```python
from build123d import *

# Parameters (mm, degrees)
SKETCH1_W           = 1.5
SKETCH1_H           = 3
BOSS_EXTRUDE1_DEPTH = 5


with BuildPart() as part:
    # Sketch1 → Boss-Extrude1 (new body)
    with BuildSketch(Plane(origin=(0, 0, 0), x_dir=(1, 0, 0), z_dir=(0, 1, 0))):
        Rectangle(SKETCH1_W, SKETCH1_H)
        Polygon((0.75, 6), (0.75, 1.5), (-0.75, 1.5), (-0.75, 7.5), (0.75, 7.5), (2.25, 6), align=None)
    extrude(amount=BOSS_EXTRUDE1_DEPTH)


solid = part.part
```
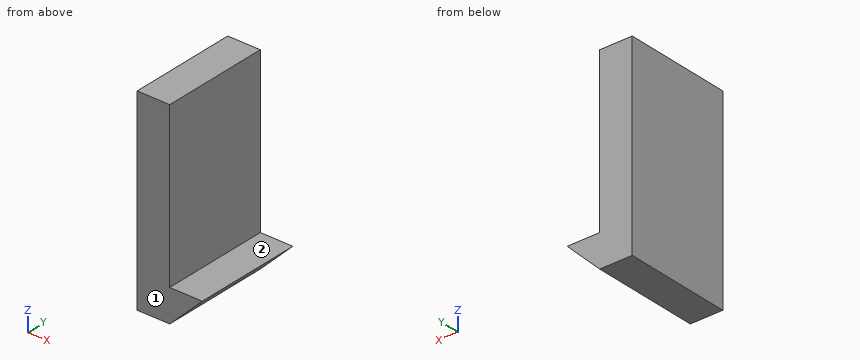
Read the model definition and answer for the solid it produces. Units are mm, in the model's axes. Face numbers are marked on the shaded views. A direction names the side the tool comes from. Coordinates: 2 decimals unless noted, no trailing zeros. Loops run counter-clockwise (first coordinate to the right, second up) from the corner with the lowest first, then second, coordinate; pieces in that order, holes last. Notation, with made-up numbers: (74.25, 10.5) -> (121.25, 10.5) arc R19 ccw to (121.25, 37.5) -> close; hole circle Ø9 at (-24, 59). An arc over 180 degrees is marked (long way). Return JSON: item names as keys, results as strings.
Item 1: Find the intervals of material crossed by probe 1 along X at (y, z) = (4.1, -3.75); probe 2 along Z at (x, y) = (1.75, 3.35); probe 3 along Z at (x, y) = (1.8, 4.1), in increasing order.
Answers:
{"probe 1": "x = -0.75 to 0.75", "probe 2": "z = -6.5 to -6", "probe 3": "z = -6.45 to -6"}
Item 2: Flat-ended cylindrical pins translate along their axes: P1, Ø1.2, axis at x = 1.5, y = 3, coming from the +Z side; P2, Ø1, axis at y = 0.5, z = -1, coming from the +X side. Find the tip coordinate at first contact, or state that the pin passes through.
Answers:
{"P1": "stops at z = -6", "P2": "stops at x = 0.75"}
Item 3: Find section B-B (x = 1.05). Determine the outline of the cut face in (y, z), plus the area to 3 significant figures.
Answers:
{"outline": "(0, -7.2) -> (5, -7.2) -> (5, -6) -> (0, -6) -> close", "area": "6.00 mm2"}
Item 4: For the marked faces 1 and 2, determine the directions among +Z, -Z, +X, -X, +Y, -Y from which every point of the face is accessible in a straight line to the end or side of a thin tool.
Answers:
{"face 1": "+Z, -Z, +X, -X, -Y", "face 2": "+Z, +X, +Y, -Y"}
Item 5: Find section C-C (z = -0.75). Determine the outline of the cut face in (x, y), plus the area to 3 significant figures.
Answers:
{"outline": "(-0.75, 0) -> (0.75, 0) -> (0.75, 5) -> (-0.75, 5) -> close", "area": "7.50 mm2"}
Item 6: Find section A-A (y = 1.6). Determine the outline of the cut face in (x, z).
Answers:
{"outline": "(-0.75, -7.5) -> (0.75, -7.5) -> (2.25, -6) -> (0.75, -6) -> (0.75, 1.5) -> (-0.75, 1.5) -> close"}
